Drawing for the job (mm, zero at the part's lowest x, y, z). Round coordinates to 2 decimals unless told otherwise and drop trailing zeros. Loops run counter-clockwise (first coordinate to the right, second up) from the corner with the lowest first, then second, coordinate; pieces in that order, holes last. Notation, with made-up numbers: M 57,28 L 95,28 A13 cw 95,46 Z; hole C -16.75,89.5 d3. An arc over 180 degrees is marked long. Answer in a Markdown table with one row per item.
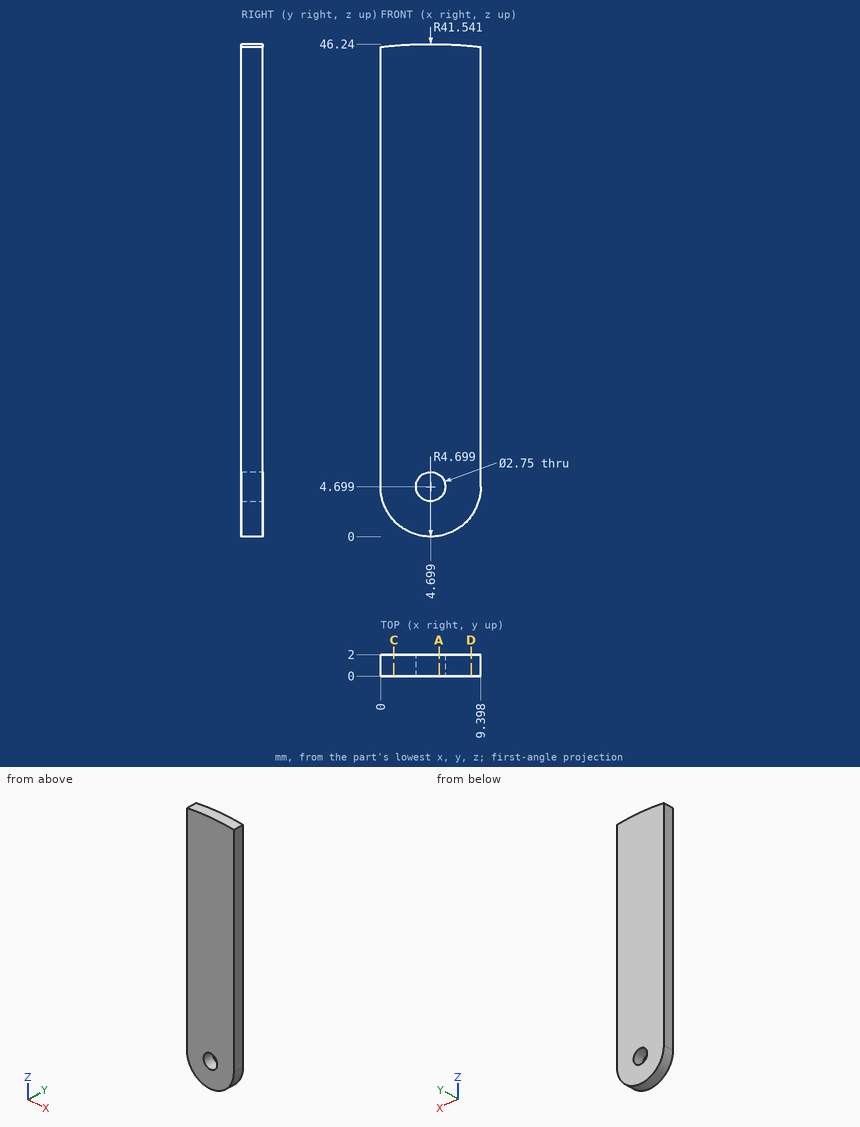
1. Pin check, flat tips, straight feed: pin 1 (1 mm diameter, centred on x = 8, y = 1, fed in from -Z) (1 decimal); pin 2 (2.5 mm diameter, centred on x = 4.699, z = 4.699, fed in from +Y); pin 3 (1 mm diameter, centred on x = 6.5, y = 1, fed in from +Z); pin 4 (1 mm diameter, centred on x = 5, z = 27.5, fed in from -Y). Stop position of each tip, or through.
Verdict:
| item | result |
|---|---|
| pin 1 | stops at z = 0.9 |
| pin 2 | passes through |
| pin 3 | stops at z = 46.22 |
| pin 4 | stops at y = 0 |
2. Wall check: probe 1 along X at (y, z) = (1.3, 4) (1 decimal); probe 2 along Z at (x, y) = (0.5, 1.1) (1 decimal); probe 3 along Z at (x, y) = (3.5, 1.1) (1 decimal). Give the ranges that are in metal, low to high.
Verdict:
| item | result |
|---|---|
| probe 1 | x = 0.1 to 3.5, 5.9 to 9.3 |
| probe 2 | z = 2.6 to 46 |
| probe 3 | z = 0.2 to 4, 5.4 to 46.2 |
3. Saw through at C-C (x = 1.25). Write the cut outline in (y, z).
Verdict:
| item | result |
|---|---|
| outline | M 0,1.51 L 2,1.51 L 2,46.1 L 0,46.1 Z |
4. Saw through at D-D (x = 8.5). Write the cut outline in (y, z).
Verdict:
| item | result |
|---|---|
| outline | M 0,1.94 L 2,1.94 L 2,46.07 L 0,46.07 Z |
5. Saw through at A-A (x = 5.5). Write the cut outline in (y, z).
Verdict:
| item | result |
|---|---|
| outline | M 0,0.07 L 2,0.07 L 2,3.58 L 0,3.58 Z; M 0,5.82 L 2,5.82 L 2,46.23 L 0,46.23 Z |
